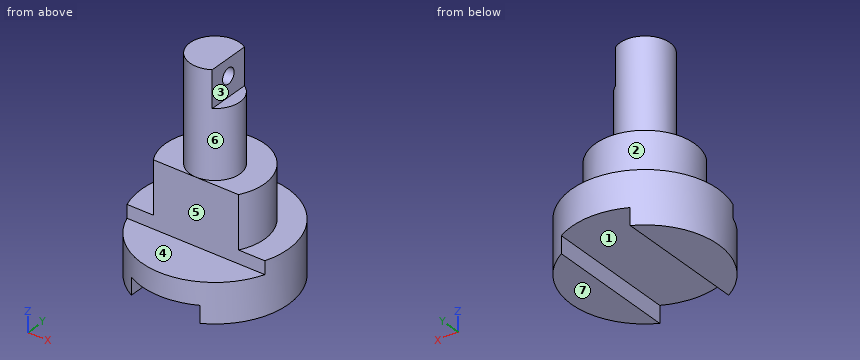
Autodesk Inventor part; units mm, degrees
ref_plane "YZ Plane" through (0, 0, 0) normal (1, 0, 0) x (0, 1, 0)
ref_plane "XZ Plane" through (0, 0, 0) normal (0, 1, 0) x (-1, 0, 0)
ref_plane "XY Plane" through (0, 0, 0) normal (0, 0, 1) x (1, 0, 0)
sketch "스케치1" plane through (0, 0, 0) normal (0, 0, 1) x (1, 0, 0)
  circle A0 centre (0, 0) radius 14.0239
extrude "돌출1" add sketch "스케치1" along normal blind 10
sketch "스케치2" plane through (0, 0, 10) normal (0, 0, 1) x (1, 0, 0)
  circle A0 centre (0, 0) radius 9.454
extrude "돌출2" add sketch "스케치2" along normal blind 10
sketch "스케치3" plane through (0, 0, 20) normal (0, 0, 1) x (1, 0, 0)
  circle A0 centre (0, 0) radius 4.783
extrude "돌출3" add sketch "스케치3" along normal blind 20
sketch "스케치4" plane through (0, 0, 40) normal (0, 0, 1) x (1, 0, 0)
  circle A0 centre (0, 0) radius 4.783
  line L0 (7.0161, -4.0466) -> (2.5499, -4.0466)
  line L1 (2.5499, -4.0466) -> (2.5499, 4.0466)
  line L2 (2.5499, 4.0466) -> (7.0161, 4.0466)
  line L3 (7.0161, 4.0466) -> (7.0161, -4.0466)
  circle A1 centre (0, 0) radius 4.783
  line L4 (7.0161, -4.0466) -> (2.5499, 4.0466) construction
  line L5 (2.5499, -4.0466) -> (7.0161, 4.0466) construction
  point P0 (4.783, 0)
extrude "돌출4" cut sketch "스케치4" against normal blind 7 contours A0 L1 | A0 L2 L3 L0 picked at (3.2943, 0)
sketch "스케치5" plane through (2.5499, -4.0466, 40) normal (1, 0, 0) x (0, 0, -1)
  circle A0 centre (3.1932, 4.0466) radius 1.4587
  point P0 (40, 4.0466)
extrude "돌출5" cut sketch "스케치5" against normal blind 7
sketch "스케치6" plane through (0, 0, 20) normal (0, 0, 1) x (1, 0, 0)
  circle A0 centre (0, 0) radius 14.0239
  line L0 (13.1762, -23.246) -> (-13.1762, -23.246)
  line L1 (-13.1762, -23.246) -> (-13.1762, -4.8019)
  line L2 (-13.1762, -4.8019) -> (13.1762, -4.8019)
  line L3 (13.1762, -4.8019) -> (13.1762, -23.246)
  line L4 (13.1762, -23.246) -> (-13.1762, -4.8019) construction
  line L5 (-13.1762, -23.246) -> (13.1762, -4.8019) construction
  point P0 (0, -14.0239)
extrude "돌출6" cut sketch "스케치6" against normal blind 12.5 contours L2 A0 | A0 L3 L0 L1 picked at (-1.1305, -9.7665)
sketch "스케치7" plane through (0, 0, 0) normal (0, 0, -1) x (-1, 0, 0)
  line L0 (6.585, 15.6352) -> (-6.585, 15.6352)
  line L1 (-6.585, 15.6352) -> (-6.585, -15.6352)
  line L2 (-6.585, -15.6352) -> (6.585, -15.6352)
  line L3 (6.585, -15.6352) -> (6.585, 15.6352)
  line L4 (6.585, 15.6352) -> (-6.585, -15.6352) construction
  line L5 (-6.585, 15.6352) -> (6.585, -15.6352) construction
  point P0 (0, 0)
extrude "돌출7" cut sketch "스케치7" against normal blind 3.25
properties part number "240628_final4"
Check sheet for the modelled part. Datum: model origin and axes. Units: mm. Face numbers are marked on the shaded views. A direction names the side the tool comes from. Coordinates: 2 decimals unless noted, no trailing zeros. Loops run counter-clockwise (first coordinate to the right, second up) from the corner with the lowest first, then second, coordinate; pieces in that order, holes last.
1) Sectioned sample at D-D (y = 11.75). Record the boundary of the cut face in (x, z) (3 decimals).
2) Sectioned sample at C-C (z = 27). Record the boundary of the cut face in (x, y).
3) Gauge pin test, flat ends, axial feed: pin 1 (1 mm diameter, centred on y = 3, z = 2.5, fed in from +X); pin 2 (6.5 mm diameter, centred on x = -2, y = -5.5, fed in from -Z); pin 3 (5.5 mm diameter, centred on x = 5.5, y = 2, fed in from +Z); pin 4 (7 mm diameter, centred on x = 3, y = 5, fed in from +Z). Record the tip position at first contact, or that the pin passes through.
4) Access from +Z, -Z, +X, -X, +Y, -Y to the whole of each face (thin tool, end or side, straight path). Record for the marked faces 5, 6 and 7.
5) Release check for a two-part mould opening along X. For the marked faces 1, 2, 3 and 4 record: released by +X, released by -X, zero draft, split by the parting line, or undercut.
6) Material ranges on probe 1 along Z at (x, y) = (11.25, -5.75); probe 2 along Z at (x, y) = (-11.75, 3.75); probe 3 along X at (y, z) = (-5.75, 3) (3 decimals), recorded low to high.
Check sheet entries:
1. outline: (-7.656, 0) - (-6.585, 0) - (-6.585, 3.25) - (6.585, 3.25) - (6.585, 0) - (7.656, 0) - (7.656, 10) - (-7.656, 10) - close
2. outline: circle Ø9.57 at (0, 0)
3. pin 1: stops at x = 13.8
3. pin 2: stops at z = 3.25
3. pin 3: stops at z = 33
3. pin 4: stops at z = 40
4. face 5: +Z, +X, -X, -Y
4. face 6: +Z
4. face 7: -Z, +X, -X, +Y, -Y
5. face 1: undercut
5. face 2: split by the parting line
5. face 3: released by +X
5. face 4: zero draft
6. probe 1: z = 0 to 7.5
6. probe 2: z = 0 to 10
6. probe 3: x = -12.791 to -6.585, 6.585 to 12.791
